Autodesk Inventor part; units mm, degrees
ref_plane "YZ Plane" through (0, 0, 0) normal (1, 0, 0) x (0, 1, 0)
ref_plane "XZ Plane" through (0, 0, 0) normal (0, 1, 0) x (-1, 0, 0)
ref_plane "XY Plane" through (0, 0, 0) normal (0, 0, 1) x (1, 0, 0)
sketch "スケッチ1" plane through (0, 0, 0) normal (0, 0, 1) x (1, 0, 0)
  circle A0 centre (0, 0) radius 2
  dimension "d0" = 4
extrude "押し出し1" add sketch "スケッチ1" along normal blind 12
sketch "スケッチ2" plane through (0, 0, 12) normal (0, 0, 1) x (1, 0, 0)
  circle A0 centre (0, 0) radius 4
  dimension "d3" = 8
extrude "押し出し2" add sketch "スケッチ2" along normal blind 2.3
chamfer "面取り1" distance 2 angle 45 1 edges at (-4, 0, 12)
sketch "スケッチ3" plane through (0, 0, 14.3) normal (0, 0, 1) x (1, 0, 0)
  line L0 (1.7321, 0) -> (0.866, -1.5)
  line L1 (0.866, -1.5) -> (-0.866, -1.5)
  line L2 (-0.866, -1.5) -> (-1.7321, 0)
  line L3 (-1.7321, 0) -> (-0.866, 1.5)
  line L4 (-0.866, 1.5) -> (0.866, 1.5)
  line L5 (0.866, 1.5) -> (1.7321, 0)
  point P0 (0, 0)
  point P1 (0, 0)
  dimension "d9" = 3
extrude "押し出し3" cut sketch "スケッチ3" against normal blind 2
thread "ねじ1"
properties part number "M4皿ネジ　12" material "鉄 灰色"
Read the model definition and answer for the solid it produces. Units are mm, in the model's axes. A direction names the side the tool comes from. Give positions to 0.01 mm unless a question says otherwise; leave off trailing zeros. Order: outer loops, then holes, each group sorted by start corner. A loop starts at its lowest first (then second) coordinate and runs counter-clockwise, first axis right, second up. Notation, with made-up numbers: (18, 11) -> (40, 11) arc R14 cw to (40, 21) -> close; hole circle Ø4 at (14.25, -36.75). An arc over 180 degrees is marked (long way). One line per item, written item: value. Start each with the question number.
(1) For a pull along Y with two mould halves and no side action, classify faces 4 (the flat face through (0, 1.5, 13)), 5 (the flat face through (0, 0, 0)), 6 (the conical face through (-0.46, -2.08, 12.13)), 7 (the flat face through (1.293, 0.76, 13.314)) as released by +Y, released by -Y, zero draft, split by the parting line, or undercut.
(2) The part is cut by section B-B (z = 1). Determine the outline of the cut face in (x, y), and give its area (3 significant figures).
(3) A tool of negligible diameter and unlimited length cuts with its end or side. For faces 1 (the flat face through (-1.293, -0.76, 13.314)), 2 (the flat face through (2, 0, 14.3)), 3 (the cylindrical face through (0, 2, 6)), from which of +Z, -Z, +X, -X, +Y, -Y can it reach the whole face along a straight path? Write none if from no direction.
(4) Flat-ended cylindrical pins translate along their axes: P1, Ø2, axis at x = -0.5, z = 4, coming from the -Y side; P2, Ø0.9, axis at x = 0, z = 13.5, coming from the +Y side; P3, Ø3, axis at x = -1, z = 6, coming from the +Y side. Find the tip coordinate at first contact, or state that the pin passes through.
(5) Straight lines are drawn through the part: L1, parallel to Y at x = 0, z = 11.5; L2, parallel to Z at x = 1, y = 0.5; L3, parallel to Z at x = -1.5, y = -3.5. For each, find the intervals that lie inside material, in ascending order.
Taken from the geometry:
1. face 4: undercut
1. face 5: zero draft
1. face 6: split by the parting line
1. face 7: undercut
2. outline: circle Ø4 at (0, 0)
2. area: 12.6 mm^2
3. face 1: +Z
3. face 2: +Z, +X, -X, +Y, -Y
3. face 3: -Z
4. P1: y = -2
4. P2: y = 3.95
4. P3: y = 2
5. L1: -2 to 2
5. L2: 0 to 12.3
5. L3: 13.81 to 14.3
